```python
from build123d import *

# Parameters (mm, degrees)
SKETCH2_W          = 12
SKETCH2_H          = 1.5
CUT_EXTRUDE3_DEPTH = 12


with BuildPart() as part:
    # Sketch2 → Revolve1 (revolve)
    with BuildSketch(Plane.XY, mode=Mode.PRIVATE) as revolve1_sk:
        Polygon((6, 1.5), (6, 0), (18, 0), (18, 27), (6, 27), align=None)
        with Locations((0, 0.75)):
            Rectangle(SKETCH2_W, SKETCH2_H)
    revolve(revolve1_sk.sketch.rotate(Axis((6, 0, 0), (-1, 0, 0)), 90), axis=Axis((6, 0, 0), (-1, 0, 0)))

    # Sketch3 → Cut-Extrude3 (cut)
    with BuildSketch(Plane(origin=(18, 0, 0), x_dir=(0, 0, -1), z_dir=(1, 0, 0))):
        Polygon((-7.194506707, 24.442263521), (-8.742565729, 29.206625443), (-10.641704711, 28.579512114), (-9.096619739, 23.824229533), align=None)
        Polygon((0.710692324, 25.469198833), (0.710669504, 30.478752832), (-1.289307676, 30.469198833), (-1.289307676, 25.469198833), align=None)
        Polygon((8.546323839, 24.003031509), (10.094339455, 28.767407535), (8.189295778, 29.37634808), (6.644210806, 24.621065498), align=None)
        Polygon((15.54538163, 20.187280222), (18.489905129, 24.240107954), (16.866273903, 25.407935699), (13.927347641, 21.362850727), align=None)
        Polygon((21.022749156, 14.395457294), (25.075550062, 17.340017716), (23.892263624, 18.952417544), (19.847178652, 16.013491283), align=None)
        Polygon((24.442263521, 7.194506707), (29.206625443, 8.742565729), (28.579512114, 10.641704711), (23.824229533, 9.096619739), align=None)
        Polygon((25.469198833, -0.710692324), (30.478752832, -0.710669504), (30.469198833, 1.289307676), (25.469198833, 1.289307676), align=None)
        Polygon((24.003031509, -8.546323839), (28.767407535, -10.094339455), (29.37634808, -8.189295778), (24.621065498, -6.644210806), align=None)
        Polygon((20.187280222, -15.54538163), (24.240107954, -18.489905129), (25.407935699, -16.866273903), (21.362850727, -13.927347641), align=None)
        Polygon((14.395457294, -21.022749156), (17.340017716, -25.075550062), (18.952417544, -23.892263624), (16.013491283, -19.847178652), align=None)
        Polygon((7.194506707, -24.442263521), (8.742565729, -29.206625443), (10.641704711, -28.579512114), (9.096619739, -23.824229533), align=None)
        Polygon((-0.710692324, -25.469198833), (-0.710669504, -30.478752832), (1.289307676, -30.469198833), (1.289307676, -25.469198833), align=None)
        Polygon((-8.546323839, -24.003031509), (-10.094339455, -28.767407535), (-8.189295778, -29.37634808), (-6.644210806, -24.621065498), align=None)
        Polygon((-15.54538163, -20.187280222), (-18.489905129, -24.240107954), (-16.866273903, -25.407935699), (-13.927347641, -21.362850727), align=None)
        Polygon((-21.022749156, -14.395457294), (-25.075550062, -17.340017716), (-23.892263624, -18.952417544), (-19.847178652, -16.013491283), align=None)
        Polygon((-24.442263521, -7.194506707), (-29.206625443, -8.742565729), (-28.579512114, -10.641704711), (-23.824229533, -9.096619739), align=None)
        Polygon((-25.469198833, 0.710692324), (-30.478752832, 0.710669504), (-30.469198833, -1.289307676), (-25.469198833, -1.289307676), align=None)
        Polygon((-24.003031509, 8.546323839), (-28.767407535, 10.094339455), (-29.37634808, 8.189295778), (-24.621065498, 6.644210806), align=None)
        Polygon((-20.187280222, 15.54538163), (-24.240107954, 18.489905129), (-25.407935699, 16.866273903), (-21.362850727, 13.927347641), align=None)
        Polygon((-14.395457294, 21.022749156), (-17.340017716, 25.075550062), (-18.952417544, 23.892263624), (-16.013491283, 19.847178652), align=None)
    extrude(amount=-CUT_EXTRUDE3_DEPTH, mode=Mode.SUBTRACT)


solid = part.part
```
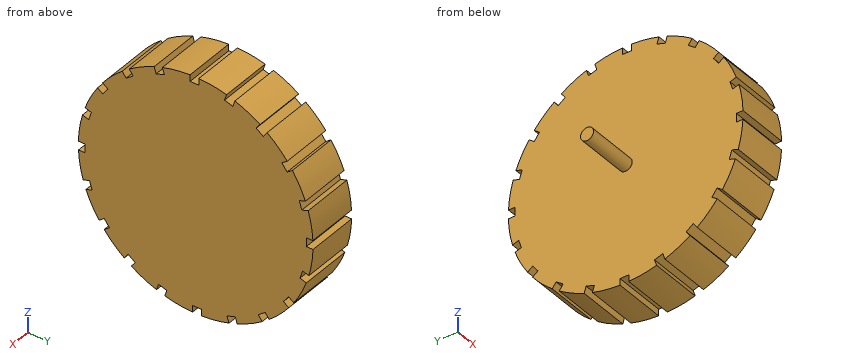
Model file for the job. Use its own axes, mm. Round coordinates to 2 decimals unless told otherwise and drop trailing zeros. Write each loop counter-clockwise with the first axis right and the second up, starting at its lowest first coordinate (ties: lowest second). Pieces come first, ordered by that corner, then holes. Notation, with made-up numbers: (-3, 36) -> (19, 36) arc R25 cw to (19, 75) -> close; hole circle Ø10 at (57, -17). An arc over 180 degrees is marked (long way). Answer as CSV lines item,"result".
1. Drill centre lines: line 1 (X direction, y = -11, z = -10.5); line 2 (Y direction, x = 15, z = -0.5); line 3 (Y direction, x = 15, z = 15). Where is each one in solid material? Low to high.
Resolved:
line 1,"6 to 18"
line 2,"-25.47 to 25.47"
line 3,"-20.58 to 20.58, 21.85 to 22.45"
2. Slice it at D-D, the plane y = -13. List the corners of the cut face in (x, z), plus the area to 3 significant figures.
Resolved:
outline,"(6, -23.66) -> (18, -23.66) -> (18, 23.66) -> (6, 23.66) -> close"
area,"568 mm²"
3. Slice it at C-C, the plane x = -2.75. List the corners of the cut face in (y, z), plus the area to 3 significant figures.
Resolved:
outline,"circle Ø3 at (0, 0)"
area,"7.07 mm²"
4. Pin check, flat tips, straight feed: pin 1 Ø1.2 at (x, y) = (9.5, -26.5) entering from +Z; pin 2 Ø8 at (x, y) = (6, -13.5) entering from +Z; pin 3 Ø10 at (y, z) = (17.5, 5) entering from -X; pin 4 Ø4 at (x, z) = (2.5, -19) entering from -Y. Stop position of each tip, or through.
Resolved:
pin 1,"z = 7.11"
pin 2,"z = 25.25"
pin 3,"x = 6"
pin 4,"through"
5. Slice it at A-A, the plane y = 0. List the corners of the cut face in (x, z).
Resolved:
outline,"(-6, -1.5) -> (6, -1.5) -> (6, -25.47) -> (18, -25.47) -> (18, 25.47) -> (6, 25.47) -> (6, 1.5) -> (-6, 1.5) -> close"
